Can you work these out from the drawing? Everything is in mm from the part's minimum corner. A direction names the side the tool comes from. Coordinates: 2 decimals unless noted, no trailing zeros. Loops run counter-clockwise (first coordinate to the right, second up) from the corner with the lowest first, then second, coordinate; pieces in that order, holes last. Notation, with made-up numbers: M 10,65.25 L 52,65.25 A20 ccw 52,104.25 Z; hole C 85.5,45.25 d8. An arc over 180 degrees is marked long. Use CSV: the item, a comma, the result in double quotes. Start each with the question number.
Q1. For pin 1 Ø4 at (x, z) = (59.85, 2.5) entering from +Y; pin 2 Ø1.2 at (x, y) = (11.5, 37) entering from -Z; pin 3 Ø13 at (y, z) = (28.5, 44) entering from -X, each with a flat end and sliding along its axis, tell me the tip position at first contact or that it passes through.
Q2. If we section it at D-D (z = 45.68): Please give me the cut outline in (x, y).
Q3. If we section it at A-A (x = 2.5): Please give me the cut outline in (y, z), and give its area (3 significant figures).
Q4. Which directions (+Z, -Z, +X, -X, +Y, -Y) give clear straight access to the entire face, cutting with the end or side of a thin tool? Please do the marked faces 1, 2 and 3.
Q5. If we section it at B-B (z = 52.18): Please give me the cut outline in (x, y), and give its area (3 significant figures).
Q6. If we section it at C-C (x = 12): Please give me the cut outline in (y, z), and give its area (3 significant figures).
Q7. Please list where these lines run through material, in increasing order: probe 1 along X at (y, z) = (5.5, 52.18); probe 2 along Z at (x, y) = (2.5, 7.25); probe 3 along Y at (x, z) = (45.5, 5). Write a range as [from, to].
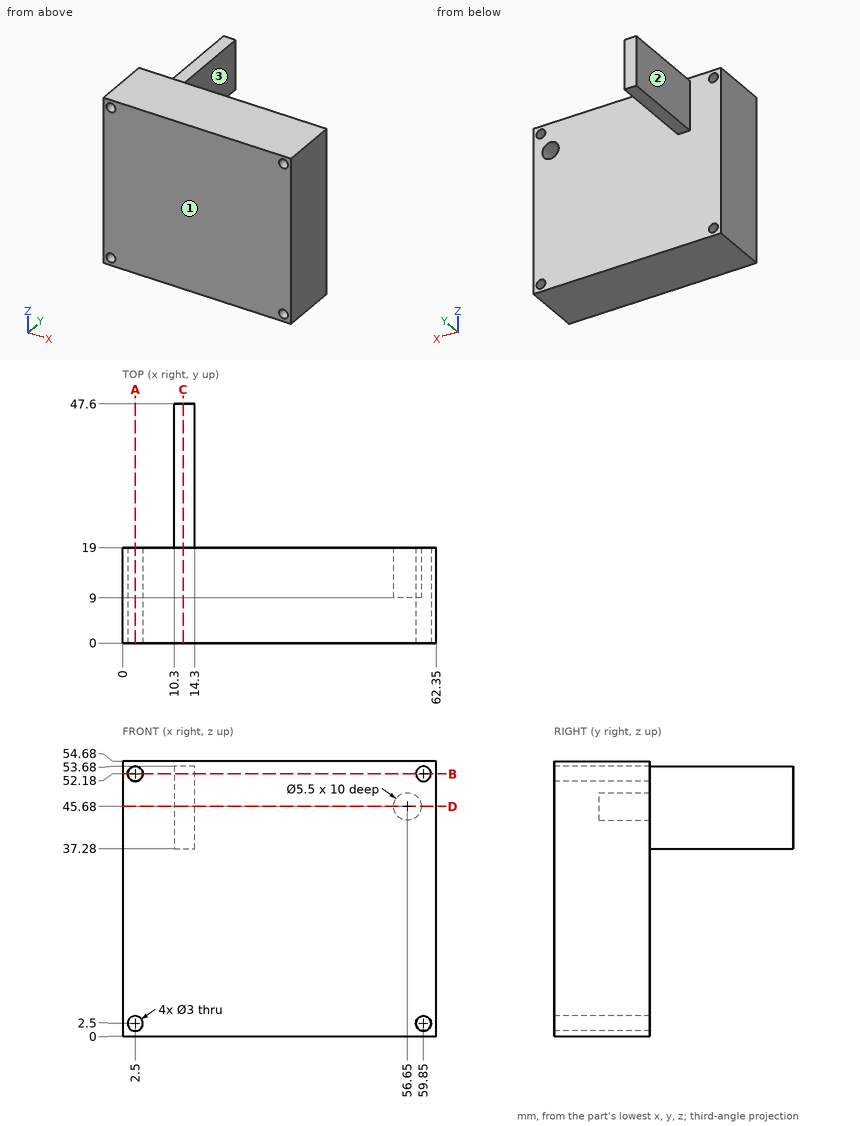
Results below:
1,pin 1,"y = 19"
1,pin 2,"z = 37.28"
1,pin 3,"x = 10.3"
2,outline,"M 0,0 L 62.35,0 L 62.35,19 L 59.4,19 L 59.4,9 L 53.9,9 L 53.9,19 L 14.3,19 L 14.3,47.6 L 10.3,47.6 L 10.3,19 L 0,19 Z"
3,outline,"M 0,0 L 19,0 L 19,1 L 0,1 Z; M 0,4 L 19,4 L 19,50.68 L 0,50.68 Z; M 0,53.68 L 19,53.68 L 19,54.68 L 0,54.68 Z"
3,area,"925 mm^2"
4,face 1,"+Z, -Z, +X, -X, -Y"
4,face 2,"+Z, -Z, -X, +Y"
4,face 3,"+Z, -Z, +X, +Y"
5,outline,"M 0,0 L 1,0 L 1,19 L 0,19 Z; M 4,0 L 58.35,0 L 58.35,19 L 14.3,19 L 14.3,47.6 L 10.3,47.6 L 10.3,19 L 4,19 Z; M 61.35,0 L 62.35,0 L 62.35,19 L 61.35,19 Z"
5,area,"1,190 mm^2"
6,outline,"M 0,0 L 19,0 L 19,37.28 L 47.6,37.28 L 47.6,53.68 L 19,53.68 L 19,54.68 L 0,54.68 Z"
6,area,"1,510 mm^2"
7,probe 1,"[0, 1], [4, 58.35], [61.35, 62.35]"
7,probe 2,"[0, 1], [4, 50.68], [53.68, 54.68]"
7,probe 3,"[0, 19]"
